from build123d import *


with BuildPart() as f1:
    # F0 (on Front) → F1 (revolve)
    with BuildSketch(Plane.XZ):
        Polygon((-19, -0.85), (19, -0.85), (19, 0.85), (-19, 0.85), (-19, 0.55), (-19, -0.55), align=None)
        Polygon((-19.5, -0.55), (-19, -0.55), (-19, 0.55), (-19.5, 0.55), (-19.5, 0.85), (-20.155381, 0.85), (-20.155381, -0.85), (-19.5, -0.85), align=None)
    revolve(axis=Axis((0, 0, -0.85), (-1, 0, 0)))


solid = f1.part
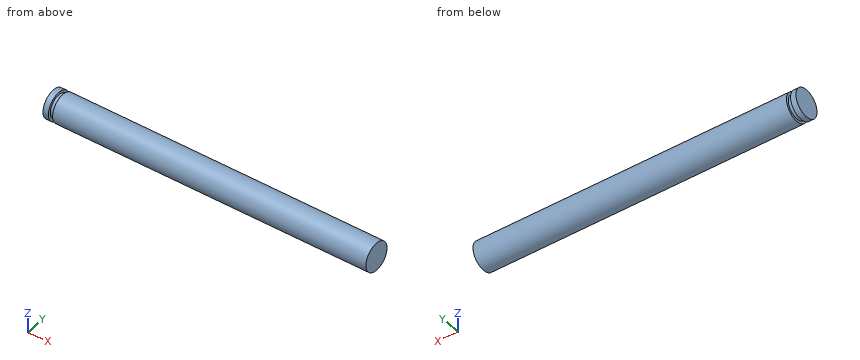
Geometry check sheet. Reference: the model listing, model coordinates, mm. Give positions to 0.01 mm unless a question says otherwise; leave off trailing zeros. Order: outer loops, then holes, each group sorted by start corner. A loop starts at its lowest first (then second) coordinate and runs counter-clockwise, first axis right, second up.
1. Depth check by flat-ended pin: pin 1 (2 mm diameter, centred on x = 14, y = 1.5, fed in from +Z); pin 2 (1.5 mm diameter, centred on x = -4, z = 0, fed in from -Y); pin 3 (1 mm diameter, centred on x = 7, y = 1.5, fed in from -Z). Enter the tip coordinate at first touch or a pass-through.
Completed:
pin 1: stops at z = 0.77
pin 2: stops at y = -1.7
pin 3: stops at z = -2.22
2. Scan lines: line 1 (X direction, y = 1.45, z = -0.15); line 2 (Y direction, x = -19.3, z = -0.85); line 3 (Z direction, x = -2, y = 0.1). Record each from-to range of solid material in increasing order.
Completed:
line 1: x = -20.16 to -19.5, -19 to 19
line 2: y = -1.4 to -0.3, 0.3 to 1.4
line 3: z = -2.55 to 0.85
3. Sectioned sample at A-A (x = 3.5). Record the boundary of the cut face in (y, z).
Completed:
outline: circle Ø3.4 at (0, -0.85)
